```python
from build123d import *

# Parameters (mm, degrees)
F1_DEPTH    = 23
F3_DEPTH    = 10
F4_R        = 0.5
F5_T1_DEPTH = 14.1433659759


# Not quite as in the source:
# - a fillet or chamfer that OpenCascade refuses, or shapes differently, is made with other operations: its cross-section is extruded or revolved along the edge and cut away or added


with BuildPart() as f1:
    # F0 (on Right) → F1 (new body)
    with BuildSketch(Plane.YZ):
        with BuildLine():
            Line((-21.5, 0), (0, 0))
            Line((0, 0), (0, 6.5))
            ThreePointArc((0, 6.5), (-0.2214821291, 8.1823237932), (-0.8708348754, 9.75))
            Line((-0.8708348754, 9.75), (-2.1698729811, 9))
            ThreePointArc((-2.1698729811, 9), (-6.5, 1.5), (-10.8301270189, 9))
            Line((-10.8301270189, 9), (-12.1291651246, 9.75))
            Line((-12.1291651246, 9.75), (-17.0941333421, 6.880740392))
            Line((-17.0941333421, 6.880740392), (-17.4823619098, 5.4318516526))
            ThreePointArc((-17.4823619098, 5.4318516526), (-18, 1.5), (-18.5176380902, 5.4318516526))
            Line((-18.5176380902, 5.4318516526), (-18.9058666579, 6.880740392))
            ThreePointArc((-18.9058666579, 6.880740392), (-20.776736691, 5.6306650015), (-21.5, 3.5))
            Line((-21.5, 3.5), (-21.5, 0))
        make_face()
    extrude(amount=F1_DEPTH)

    # F2 (on face) → F3 (join)
    with BuildSketch(Plane.XZ.offset(21.5)):
        Polygon((3, 0), (0, 0), (0, -10.9), (13, -10.9), (13, -7.9), (3, -7.9), align=None)
    extrude(amount=-F3_DEPTH)

    # F4
    f4_edges = [f1.edges().sort_by_distance(p)[0] for p in [
        (0, -18, 1.5),
        (0, -17.288248, 6.156296),
        (0, -14.611649, 8.31537),
        (0, -11.479646, 9.375),
        (0, -6.5, 1.5),
        (0, -1.520354, 9.375),
        (0, 0, 3.25),
        (0, -5.75, 0),
        (0, -11.5, -5.45),
        (0, -16.5, -10.9),
        (0, -21.5, -3.7),
        (0, -18.711752, 6.156296),
        (6.5, -21.5, -10.9),
        (6.5, -11.5, -10.9),
        (13, -16.5, -10.9),
        (13, -11.5, -9.4),
        (13, -21.5, -9.4),
        (11.5, -17.482362, 5.431852),
        (11.5, -17.094133, 6.88074),
        (11.5, -18.517638, 5.431852),
        (11.5, -18.905867, 6.88074),
        (11.5, -12.129165, 9.75),
        (11.5, -10.830127, 9),
        (11.5, -2.169873, 9),
        (11.5, -0.870835, 9.75),
        (0, -20.776737, 5.630665),
        (0, -0.221482, 8.182324),
    ]]
    fillet(f4_edges, radius=F4_R)

    # F5: chamfer of 1 on 1 edges, made by hand

    # F5_s2 → F5_t1 (cut)
    with BuildSketch(Plane.XZ.offset(9.428317012)):
        Polygon((12, -7.9), (13, -8.9), (13, -7.9), align=None)
    extrude(amount=F5_T1_DEPTH, mode=Mode.SUBTRACT)


solid = f1.part
```
Geometry: final body of the model. Coordinates: model frame, mm. A direction names the side the tool comes from. Round coordinates to 2 decimals unless told otherwise and drop trailing zeros. Write each loop counter-clockwise with the first axis right and the second up, starting at its lowest first coordinate (ties: lowest second). Pieces come first, ordered by that corner, then holes. Notation, with made-up numbers: (-33.75, 37) -> (-19.75, 37) arc R33 cw to (-19.75, 69) -> close; hole circle Ø5 at (28.5, -2.75). An arc over 180 degrees is marked (long way). Use CSV: the item, a comma, the result in double quotes. Start each with the question number.
Q1. Section B-B (x = 6.25). Return loops of the section in (y, z), plus the area to 3 significant figures.
Q2. First-contact query: pin 1 Ø6 at (y, z) = (-4, 3) entering from +X; pin 2 Ø1.6 at (y, z) = (-17.5, -9.5) entering from +X; pin 3 Ø9 at (y, z) = (-6.5, 6.5) entering from +X; pin 4 Ø1.5 at (x, y) = (13.5, -14.5) entering from +Z. Flat tips, straight axial feed; report the tip coordinate or a pass-through.
Q3. Reachability of faces 1 (the face through (12.5, -16.4, -8.4)), 2 (the face through (13, -17, -10)), 3 (the face through (11.592, -17.255, 6.279)), 4 (the face through (4, -11.5, -9)) from +Z, -Z, +X, -X, +Y, -Y: full face, straight path, thin tool, end or side. Return the list, or none.
Q4. Line query: L1, parallel to Y at x = 9, z = 3.5; L2, parallel to Y at x = 18.25, z = 6.5; L3, parallel to Z at x = 13, y = -6.5. Output: solid intervals per line, ascending.
Q5. Section C-C (z = 4). Give the number of separate pieces and of enclosed holes in the cut face, plus the area to 3 significant figures.
Q6. Section D-D (x = 14.25). Return loops of the section in (y, z).
Q7. Pull-direction query (Y, two-part tool) for faces 5 (the face through (11.59, -17.93, 1.5)), 6 (the face through (12, 0, 3)), 7 (the face through (11.592, -20.93, 5.414)); classes: pulls with the +Y half, pulls with the -Y half, needs draft (parallel to the pull), parting line crosses it, or undercut.
Q8. Section A-A (y = -18). Return loops of the section in (x, z).
Result sheet:
1,outline,"(-21.5, -10.4) arc R0.5 ccw to (-21, -10.9) -> (-12, -10.9) arc R0.5 ccw to (-11.5, -10.4) -> (-11.5, -7.9) -> (-21.5, -7.9) -> close; (-21.5, 0) -> (0, 0) -> (0, 6.5) arc R6.5 ccw to (-0.62, 9.27) arc R0.5 ccw to (-1.32, 9.49) -> (-1.76, 9.24) arc R0.5 ccw to (-1.96, 8.6) arc R5 cw (long way) to (-11.04, 8.6) arc R0.5 ccw to (-11.24, 9.24) -> (-11.88, 9.61) arc R0.5 ccw to (-12.38, 9.61) -> (-16.91, 6.98) arc R0.5 ccw to (-17.15, 6.68) -> (-17.37, 5.87) arc R0.5 ccw to (-17.11, 5.29) arc R2 cw (long way) to (-18.89, 5.29) arc R0.5 ccw to (-18.63, 5.87) -> (-18.77, 6.36) arc R0.5 ccw to (-19.46, 6.68) arc R3.5 ccw to (-21.5, 3.5) -> close"
1,area,"131 mm²"
2,pin 1,"x = 23"
2,pin 2,"x = 13"
2,pin 3,"through"
2,pin 4,"z = 8.81"
3,face 1,"+X, +Y, -Y"
3,face 2,"-Z, +X, +Y, -Y"
3,face 3,"+Z, +X, -X"
3,face 4,"-Z, +X, -X, +Y"
4,L1,"-21.5 to -20, -16 to -10.5, -2.5 to 0"
4,L2,"-19.8 to -18.83, -17.2 to -11.5, -1.5 to 0"
4,L3,"0 to 1.5"
5,separate pieces,"3"
5,enclosed holes,"0"
5,area,"205 mm²"
6,outline,"(-21.5, 0) -> (0, 0) -> (0, 6.5) arc R6.5 ccw to (-0.62, 9.27) arc R0.5 ccw to (-1.32, 9.49) -> (-1.76, 9.24) arc R0.5 ccw to (-1.96, 8.6) arc R5 cw (long way) to (-11.04, 8.6) arc R0.5 ccw to (-11.24, 9.24) -> (-11.88, 9.61) arc R0.5 ccw to (-12.38, 9.61) -> (-16.91, 6.98) arc R0.5 ccw to (-17.15, 6.68) -> (-17.37, 5.87) arc R0.5 ccw to (-17.11, 5.29) arc R2 cw (long way) to (-18.89, 5.29) arc R0.5 ccw to (-18.63, 5.87) -> (-18.77, 6.36) arc R0.5 ccw to (-19.46, 6.68) arc R3.5 ccw to (-21.5, 3.5) -> close"
7,face 5,"undercut"
7,face 6,"pulls with the +Y half"
7,face 7,"pulls with the -Y half"
8,outline,"(0, -10.4) arc R0.5 ccw to (0.5, -10.9) -> (12.5, -10.9) arc R0.5 ccw to (13, -10.4) -> (13, -8.9) -> (12, -7.9) -> (3, -7.9) -> (3, 0) -> (23, 0) -> (23, 1.5) -> (0.5, 1.5) arc R0.5 ccw to (0, 1) -> close"
